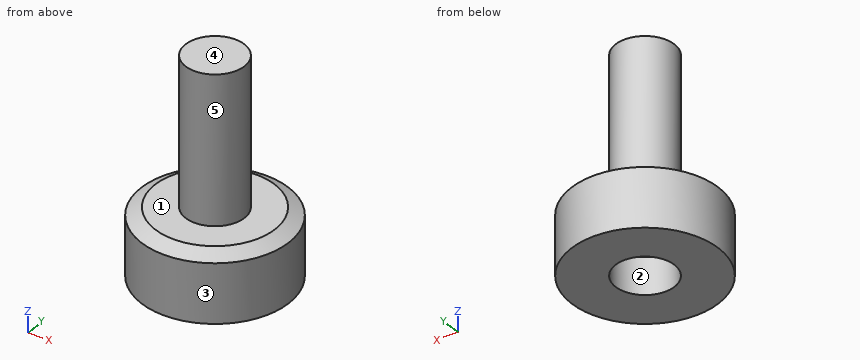
from build123d import *

# Parameters (mm, degrees)
F0_W   = 4
F0_H   = 20
F0_H_2 = 3
F0_H_3 = 1.0746234533


with BuildPart() as f1:
    # F0 (on Front) → F1 (revolve)
    with BuildSketch(Plane.XZ):
        with Locations((-22.5513077103, 19.0746234533)):
            Rectangle(F0_W, F0_H)
        Polygon((-24.5513077103, 8), (-30.5513077103, 8), (-30.5513077103, 0), (-24.5513077103, 0), (-24.5513077103, 5), align=None)
        Polygon((-28.6900052902, 9.0746234533), (-30.5513077103, 8), (-24.5513077103, 8), (-24.5513077103, 9.0746234533), align=None)
        with Locations((-22.5513077103, 6.5)):
            Rectangle(F0_W, F0_H_2)
        with Locations((-22.5513077103, 8.5373117267)):
            Rectangle(F0_W, F0_H_3)
    revolve(axis=Axis((-20.5513077103, 0, 19.0746234533), (0, 0, 1)))


solid = f1.part
Geometry: final body of the model. Coordinates: model frame, mm. Face numbers are marked on the shaded views. A direction names the side the tool comes from. Coordinates: 2 decimals unless noted, no trailing zeros. Loops run counter-clockwise (first coordinate to the right, second up) from the corner with the lowest first, then second, coordinate; pieces in that order, holes last. Notation, with made-up numbers: (24.25, 44) - (81.25, 44) arc R30 ccw to (81.25, 74) - close; hole circle Ø7 at (78.5, 21). An arc over 180 degrees is marked (long way). Put each result on its own line as item: value. Start each with the question number.
Q1. Pull-direction query (X, two-part tool) for the marked faces 1, 2 and 3; classes: released by +X, released by -X, zero draft, split by the parting line, or undercut.
Q2. Cut plane C-C, the plane z = 15.5. Return loops of the section in (x, y), and give its area (3 significant figures).
Q3. Pin query (flat end, axial travel): pin 1 Ø8 at (x, y) = (-13, 0) entering from -Z; pin 2 Ø12 at (x, z) = (-25.5, 18.5) entering from +Y; pin 3 Ø2 at (y, z) = (-7.5, 10.5) entering from +X (3 decimals); pin 4 Ø8 at (y, z) = (-7, 4) entering from +X. Return the tip coordinate at first contact, or that it passes through.
Q4. Cut plane A-A, the plane z = 4.5. Return loops of the section in (x, y), and give its area (3 significant figures).
Q5. Set-up query: the marked faces 4 and 5. Return all of +Z, -Z, +X, -X, +Y, -Y with unobstructed straight access to the full face (end or side cutting, diameter ignored); none if empty.
Q6. Cut plane B-B, the plane y = 0. Return loops of the section in (x, z), and give its area (3 significant figures).
Q7. Line query: line 1 (X direction, y = 0, z = 3.8); line 2 (Z direction, x = -16.5, y = -3.75); line 3 (X direction, y = 0.25, z = 13). Output: solid intervals per line, ascending.
Filled sheet:
1. face 1: zero draft
1. face 2: undercut
1. face 3: split by the parting line
2. outline: circle Ø8 at (-20.55, 0)
2. area: 50.3 mm²
3. pin 1: z = 0
3. pin 2: y = 4
3. pin 3: through
3. pin 4: x = -11.01
4. outline: circle Ø20 at (-20.55, 0); hole circle Ø8 at (-20.55, 0)
4. area: 264 mm²
5. face 4: +Z, +X, -X, +Y, -Y
5. face 5: +Z
6. outline: (-30.55, 0) - (-24.55, 0) - (-24.55, 5) - (-16.55, 5) - (-16.55, 0) - (-10.55, 0) - (-10.55, 8) - (-12.41, 9.07) - (-16.55, 9.07) - (-16.55, 29.07) - (-24.55, 29.07) - (-24.55, 9.07) - (-28.69, 9.07) - (-30.55, 8) - close
6. area: 299 mm²
7. line 1: -30.55 to -24.55, -16.55 to -10.55
7. line 2: 0 to 9.07
7. line 3: -24.54 to -16.56
